Source: CAD feature listing. Evaluate the final solid. Frame: model axes, mm. Face numbers are marked on the shaded views. A direction names the side the tool comes from. Give positions to 0.01 mm unless a question says otherwise; leave off trailing zeros. Write each loop counter-clockwise with the first axis right and the second up, starting at its lowest first coordinate (ties: lowest second). Pieces come first, ordered by that corner, then holes. Notation, with made-up numbers: (-12.5, 75) - (42.5, 75) arc R21 ccw to (42.5, 112) - close; hole circle Ø8 at (39, 49). An arc over 180 degrees is marked (long way). Answer as a JSON object with one key per item and string values. Group by question number.
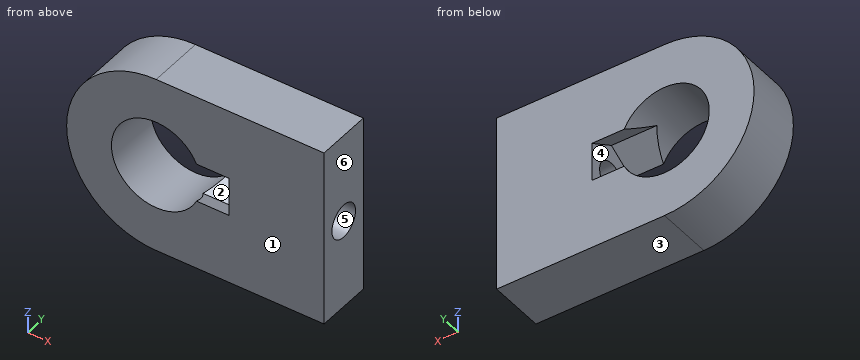
from build123d import *

# Parameters (mm, degrees)
SKETCH1_R               = 4
BOSS_EXTRUDE1_DEPTH     = 5
CUT_EXTRUDE1_REACH      = 26.86
CUT_EXTRUDE1_END_RADIUS = 4
SKETCH2_R               = 1.5
CUT_EXTRUDE2_START      = -12.56758
SKETCH2_4_R             = 1.5
CUT_EXTRUDE2_DEPTH      = 4.06758


with BuildPart() as part:
    # Sketch1 → Boss-Extrude1 (new body)
    with BuildSketch(Plane(origin=(0, 0, 0), x_dir=(1, 0, 0), z_dir=(0, 1, 0))):
        with BuildLine():
            Line((0, 8), (15, 8))
            Line((15, 8), (15, -8))
            Line((15, -8), (0, -8))
            ThreePointArc((0, -8), (-8, 0), (0, 8))
        make_face()
        with Locations(Location((0, 0, 0), (0, 0, 270))):
            Circle(SKETCH1_R, mode=Mode.SUBTRACT)
    extrude(amount=BOSS_EXTRUDE1_DEPTH)

    # Cut-Extrude1: up to this cylinder (the profile starts outside it)
    cut_extrude1_end = Plane(origin=(0, 2.5, 0), z_dir=(0, -1, 0)) * Cylinder(CUT_EXTRUDE1_END_RADIUS, 62.72, mode=Mode.PRIVATE)
    # Sketch2 → Cut-Extrude1 (cut, up to the surface)
    with BuildSketch(Plane(origin=(15, 0, 0), x_dir=(0, 0, -1), z_dir=(1, 0, 0)), mode=Mode.PRIVATE) as cut_extrude1_sk1:
        with Locations((0, 2.5)):
            Circle(SKETCH2_R)
    cut_extrude1_tool1 = extrude(cut_extrude1_sk1.sketch, amount=-CUT_EXTRUDE1_REACH, mode=Mode.PRIVATE) - cut_extrude1_end
    add(cut_extrude1_tool1.solids().sort_by_distance((15, 2.5, 0))[0], mode=Mode.SUBTRACT)

    # Sketch2_4 → Cut-Extrude2 (cut)
    with BuildSketch(Plane(origin=(15, 0, 0), x_dir=(0, 0, -1), z_dir=(1, 0, 0)).offset(CUT_EXTRUDE2_START)):
        Polygon((3.175426481, 2.5), (1.58771324, 5.25), (-1.58771324, 5.25), (-3.175426481, 2.5), (-1.58771324, -0.25), (1.58771324, -0.25), align=None)
        with Locations((0, 2.5)):
            Circle(SKETCH2_4_R, mode=Mode.SUBTRACT)
    extrude(amount=CUT_EXTRUDE2_DEPTH, mode=Mode.SUBTRACT)


solid = part.part
Q1. Reachability of the marked faces 4, 5 and 6 from +Z, -Z, +X, -X, +Y, -Y: full face, straight path, thin tool, end or side. Return the list, or none.
Q2. Section D-D on x = -3.25. Return the cut outline in (y, z), then the cut area to 3 significant figures.
Q3. Section B-B on x = 0.5. Return the cut outline in (y, z).
Q4. First-contact query: pin 1 Ø1 at (y, z) = (3, 0) entering from +X; pin 2 Ø1 at (y, z) = (1.5, 2.5) entering from -X; pin 3 Ø2 at (x, y) = (-3, 1) entering from +Z. Flat tips, straight axial feed; report the tip coordinate or a pass-through.
Q5. Ray query, probe 1 along Y at (x, z) = (10, 0); probe 2 along Z at (x, y) = (10.75, 1.8); probe 3 along X at (y, z) = (2.15, 2.5). Return the intervals inside material, ascending. Write a range as [from, to].
Q6. Section A-A on z = 0. Return the cut outline in (x, y).
Q7. Section C-C on y = 4.65. Return the cut outline in (x, z), then the cut area to 3 significant figures.
Q8. Draft query along Y for the marked faces 1, 2 and 3. Return one class per face: released by +Y, released by -Y, zero draft, split by the parting line, or undercut.
Taken from the geometry:
{
 "1": {"face 4": "none", "face 5": "+X", "face 6": "+Z, -Z, +X, +Y, -Y"},
 "2": {"outline": "(0, -7.31) - (5, -7.31) - (5, -2.33) - (0, -2.33) - close; (0, 2.33) - (5, 2.33) - (5, 7.31) - (0, 7.31) - close", "area": "49.8 mm²"},
 "3": {"outline": "(0, -8) - (5, -8) - (5, -3.97) - (0, -3.97) - close; (0, 3.97) - (5, 3.97) - (5, 8) - (0, 8) - close"},
 "4": {"pin 1": "stops at x = -3.97", "pin 2": "stops at x = -7.75", "pin 3": "stops at z = 7.75"},
 "5": {"probe 1": "y = [0, 1], [4, 5]", "probe 2": "z = [-8, -1.33], [1.33, 8]", "probe 3": "x = [-7.6, -3.12], [6.5, 15]"},
 "6": {"outline": "(-8, 0) - (-4, 0) - (-4, 5) - (-8, 5) - close; (6.5, 0) - (15, 0) - (15, 1) - (6.5, 1) - close; (6.5, 4) - (15, 4) - (15, 5) - (6.5, 5) - close"},
 "7": {"outline": "(0, -8) - (15, -8) - (15, 8) - (0, 8) arc R8 ccw to start; hole (3.5, -1.93) - (6.5, -1.93) - (6.5, 1.93) - (3.5, 1.93) arc R4 ccw (long way) to start", "area": "280 mm²"},
 "8": {"face 1": "released by -Y", "face 2": "undercut", "face 3": "zero draft"}
}
